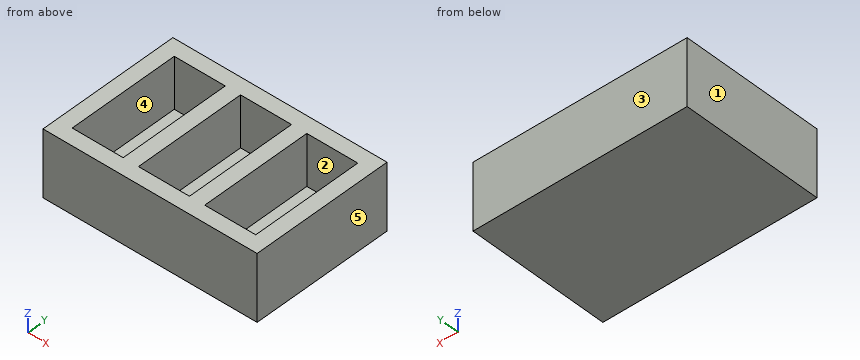
```python
from build123d import *

# Parameters (mm, degrees)
BOX004_W     = 10
BOX004_H     = 22
BOX004_DEPTH = 10
BOX003_W     = 10
BOX003_H     = 22
BOX003_DEPTH = 10
BOX002_W     = 10
BOX002_H     = 22
BOX002_DEPTH = 10
BOX001_W     = 42
BOX001_H     = 28
BOX001_DEPTH = 13


with BuildPart() as cubo003:
    # Box004 → Box004 (new body)
    with BuildSketch(Plane(origin=(29, 3, 3), x_dir=(1, 0, 0), z_dir=(0, 0, 1))):
        with Locations((5, 11)):
            Rectangle(BOX004_W, BOX004_H)
    extrude(amount=BOX004_DEPTH)


with BuildPart() as cubo002:
    # Box003 → Box003 (new body)
    with BuildSketch(Plane(origin=(16, 3, 3), x_dir=(1, 0, 0), z_dir=(0, 0, 1))):
        with Locations((5, 11)):
            Rectangle(BOX003_W, BOX003_H)
    extrude(amount=BOX003_DEPTH)


with BuildPart() as cubo001:
    # Box002 → Box002 (new body)
    with BuildSketch(Plane(origin=(3, 3, 3), x_dir=(1, 0, 0), z_dir=(0, 0, 1))):
        with Locations((5, 11)):
            Rectangle(BOX002_W, BOX002_H)
    extrude(amount=BOX002_DEPTH)


with BuildPart() as cut002:
    # Box001 → Box001 (new body)
    with BuildSketch(Plane.XY):
        with Locations((21, 14)):
            Rectangle(BOX001_W, BOX001_H)
    extrude(amount=BOX001_DEPTH)

    # Cut: cut Cubo001
    add(cubo001.part, mode=Mode.SUBTRACT)

    # Cut001: cut Cubo002
    add(cubo002.part, mode=Mode.SUBTRACT)

    # Cut002: cut Cubo003
    add(cubo003.part, mode=Mode.SUBTRACT)


solid = cut002.part
```
Input: part model. Units: mm. Frame: model coordinates. Face numbers are marked on the shaded views. A direction names the side the tool comes from. Give positions to 0.01 mm unless a question says otherwise; leave off trailing zeros. Order: outer loops, then holes, each group sorted by start corner. A loop starts at its lowest first (then second) coordinate and runs counter-clockwise, first axis right, second up.
1. Reachability of the marked faces 1 and 2 from +Z, -Z, +X, -X, +Y, -Y: full face, straight path, thin tool, end or side. Return the list, or none.
Derived:
face 1: +Z, -Z, -X, +Y, -Y
face 2: +Z
2. Section C-C on y = 19. Return the cut outline in (x, z).
Derived:
outline: (0, 0) - (42, 0) - (42, 13) - (39, 13) - (39, 3) - (29, 3) - (29, 13) - (26, 13) - (26, 3) - (16, 3) - (16, 13) - (13, 13) - (13, 3) - (3, 3) - (3, 13) - (0, 13) - close
3. Pin query (flat end, axial travel): pin 1 (8 mm diameter, centred on x = 11, y = 23.5, fed in from +Z); pin 2 (5 mm diameter, centred on x = 32, y = 19, fed in from +Z). Return the tip coordinate at first contact, or that it passes through.
Derived:
pin 1: stops at z = 13
pin 2: stops at z = 3
4. Section A-A on z = 7.5. Return the cut outline in (x, y), and give its area (3 significant figures).
Derived:
outline: (0, 0) - (42, 0) - (42, 28) - (0, 28) - close; hole (3, 3) - (13, 3) - (13, 25) - (3, 25) - close; hole (16, 3) - (26, 3) - (26, 25) - (16, 25) - close; hole (29, 3) - (39, 3) - (39, 25) - (29, 25) - close
area: 516 mm2
5. Section B-B on x = 31. Return the cut outline in (y, z), and give its area (3 significant figures).
Derived:
outline: (0, 0) - (28, 0) - (28, 13) - (25, 13) - (25, 3) - (3, 3) - (3, 13) - (0, 13) - close
area: 144 mm2
6. Material intervals for L1, parallel to X at y = 24.75, z = 11.75; L2, parallel to Y at x = 20.5, z = 7.5; L3, parallel to Z at x = 38, y = 12.25, sorted ascending.
Derived:
L1: x = 0 to 3, 13 to 16, 26 to 29, 39 to 42
L2: y = 0 to 3, 25 to 28
L3: z = 0 to 3
7. Mould query, pull axis X, two halves, no side actions, for the marked faces 3, 4 and 5. Classes: released by +X, released by -X, zero draft, split by the parting line, or undercut.
Derived:
face 3: zero draft
face 4: undercut
face 5: released by +X
